Input: part model. Units: mm. Frame: model coordinates. Give positions to 0.01 mm unless a question says otherwise; leave off trailing zeros. Loops run counter-clockwise (first coordinate to the right, second up) from the corner with the lowest first, then second, coordinate; pieces in that order, holes last. Notation, with made-up numbers: (-15, 52) - (-7, 52) arc R18 ccw to (-7, 68) - close; hole circle Ø3 at (0.5, 11). An arc over 180 degrees is marked (long way). One line per item, written item: value.
from build123d import *

# Parameters (mm, degrees)
SKIZZE1_R                       = 7.5
AUFSATZ_LINEAR_AUSTRAGEN1_DEPTH = 8
SCHNITT_LINEAR_AUSTRAGEN1_DEPTH = 9
KREISMUSTER1_COUNT              = 10
SCHNITT_LINEAR_AUSTRAGEN3_REACH = 10


with BuildPart() as part:
    # Skizze1 → Aufsatz-Linear austragen1 (new body)
    with BuildSketch(Plane.XY):
        Circle(SKIZZE1_R)
    extrude(amount=AUFSATZ_LINEAR_AUSTRAGEN1_DEPTH)

    # Skizze3 → Schnitt-Linear austragen1 (cut, through all)
    with BuildSketch(Plane.XY.offset(8)):
        with BuildLine():
            ThreePointArc((1.98549644, 4.239169305), (1.299374701, 4.497152198), (0.581391256, 4.644861324))
            ThreePointArc((0.581391256, 4.644861324), (0.684746364, 6.178122942), (-0.100097626, 7.499332001))
            ThreePointArc((-0.100097626, 7.499332001), (2.076040858, 7.20694487), (4.074246256, 6.296865684))
            ThreePointArc((4.074246256, 6.296865684), (2.704090414, 5.598714906), (1.98549644, 4.239169305))
        make_face()
    schnitt_linear_austragen1 = extrude(amount=-SCHNITT_LINEAR_AUSTRAGEN1_DEPTH, mode=Mode.SUBTRACT)

    # Kreismuster1: Schnitt-Linear austragen1 ×10 about axis
    kreismuster1_axis = Axis((0, 0, 0), (0, 0, 1))
    for i in range(1, KREISMUSTER1_COUNT):
        add(schnitt_linear_austragen1.rotate(kreismuster1_axis, i * 360 / KREISMUSTER1_COUNT), mode=Mode.SUBTRACT)

    # Skizze4 → Schnitt-Linear austragen3 (cut, up to next)
    with BuildSketch(Plane.XY.offset(8), mode=Mode.PRIVATE) as schnitt_linear_austragen3_sk1:
        with BuildLine():
            Line((1.754992877, -1.85), (-1.754992877, -1.85))
            ThreePointArc((-1.754992877, -1.85), (-2.55, 0), (-1.754992877, 1.85))
            Line((-1.754992877, 1.85), (1.754992877, 1.85))
            ThreePointArc((1.754992877, 1.85), (2.55, 0), (1.754992877, -1.85))
        make_face()
    schnitt_linear_austragen3_tool1 = extrude(schnitt_linear_austragen3_sk1.sketch, amount=-SCHNITT_LINEAR_AUSTRAGEN3_REACH, mode=Mode.PRIVATE) & part.part
    add(schnitt_linear_austragen3_tool1.solids().sort_by_distance((0, 0, 8))[0], mode=Mode.SUBTRACT)


solid = part.part
Item 1: Material intervals for L1, parallel to Y at x = -4, z = 4.5; L2, parallel to X at y = -5.5, z = 3; L3, parallel to X at y = 5.75, z = 1.25, sorted ascending.
Verdict:
L1: y = -6.28 to -4.23, -2.43 to 2.43, 3.63 to 5.91
L2: x = -4.38 to -2.61, -0.75 to 1.13, 3.2 to 4.76
L3: x = -4.74 to -3.6, -1.14 to 0.75, 2.87 to 4.38
Item 2: Pin query (flat end, axial travel): P1, Ø4, axis at y = -4.5, z = 1, coming from the -X side; P2, Ø1.1, axis at x = 0, z = 2.5, coming from the -Y side; P3, Ø4, axis at y = 3.5, z = 5.5, coming from the -X side; P4, Ø3, axis at y = -0.5, z = 6, coming from the -X side. Return the tip coordinate at first contact, or that it passes through.
Verdict:
P1: stops at x = -7.07
P2: stops at y = -7.5
P3: stops at x = -7.25
P4: stops at x = -6.87
Item 3: Section D-D, the plane y = -5. Output: boundary loops of the cut face in (x, z).
Verdict:
outline: (-4.32, 0) - (-2.25, 0) - (-2.25, 8) - (-4.32, 8) - close; (-0.69, 0) - (1.04, 0) - (1.04, 8) - (-0.69, 8) - close; (2.7, 0) - (4.72, 0) - (4.72, 8) - (2.7, 8) - close
Item 4: Section C-C, the plane x = 1.5. Output: boundary loops of the cut face in (y, z), and give its area (3 significant figures).
Verdict:
outline: (-4.43, 0) - (-1.85, 0) - (-1.85, 8) - (-4.43, 8) - close; (1.85, 0) - (4.43, 0) - (4.43, 8) - (1.85, 8) - close
area: 41.3 mm^2
Item 5: Section B-B, the plane x = 5.5. Output: boundary loops of the cut face in (y, z), and give its area (3 significant figures).
Verdict:
outline: (-2.54, 0) - (-0.61, 0) - (-0.61, 8) - (-2.54, 8) - close; (0.99, 0) - (2.94, 0) - (2.94, 8) - (0.99, 8) - close
area: 31.1 mm^2
Item 6: Section A-A, the plane y = 5.5. Output: boundary loops of the cut face in (x, z), and give its area (3 significant figures).
Verdict:
outline: (-4.76, 0) - (-3.2, 0) - (-3.2, 8) - (-4.76, 8) - close; (-1.13, 0) - (0.75, 0) - (0.75, 8) - (-1.13, 8) - close; (2.61, 0) - (4.38, 0) - (4.38, 8) - (2.61, 8) - close
area: 41.7 mm^2
Item 7: Draft query along Y for faces 1 (the face through (3, 0, 8)), 2 (the face through (-4.18, -4.58, 4.06)). Return one class per face: pulls with the +Y half, pulls with the -Y half, needs draft (parallel to the pull), parting line crosses it, or undercut.
Verdict:
face 1: needs draft
face 2: undercut
